from build123d import *

# Parameters (mm, degrees)
ESQUISSE1_R        = 13.55
ESQUISSE1_R_2      = 12.55
BOSS_EXTRU_1_DEPTH = 20
CONG_1_R           = 10
CONG_2_R           = 5


with BuildPart() as part:
    # Esquisse1 → Boss.-Extru.1 (new body)
    with BuildSketch(Plane.XY):
        Circle(ESQUISSE1_R)
        Circle(ESQUISSE1_R_2, mode=Mode.SUBTRACT)
    extrude(amount=BOSS_EXTRU_1_DEPTH)

    # Esquisse2 → Révolution1 (revolve)
    with BuildSketch(Plane(origin=(0, 0, 0), x_dir=(0, 0, -1), z_dir=(1, 0, 0)), mode=Mode.PRIVATE) as r_volution1_sk:
        with BuildLine():
            Line((18.986494144, 0), (0, 0))
            Line((0, 0), (0, -18.986494144))
            ThreePointArc((0, -18.986494144), (13.42547876, -13.42547876), (18.986494144, 0))
        make_face()
    revolve(r_volution1_sk.sketch.rotate(Axis((0, 0, -18.986494144), (0, 0, 1)), 270), axis=Axis((0, 0, -18.986494144), (0, 0, 1)))

    # Congé1
    # the kernel refuses this fillet: 10 mm, written as the material it adds along each edge
    with BuildSketch(Plane(origin=(0, 0, 0), x_dir=(1, 0, 0), z_dir=(0, -1, 0))) as cong_1_piece_1:
        with BuildLine():
            CenterArc((23.55, 8.898000579), CONG_1_R, 180, 62.848132995)
            Line((13.55, 8.898000579), (13.35, 8.898000579))
            Line((13.35, 8.898000579), (13.35, 0))
            Line((13.35, 0), (13.55, -0.2))
            ThreePointArc((13.55, -0.2), (16.268247072, -0.2), (18.895224027, -0.177960012))
            Line((18.895224027, -0.177960012), (18.986494144, 0))
        make_face()
    revolve(axis=Axis((0, 0, 0), (0, 0, 1)))

    # Congé2
    cong_2_edges = [part.edges().sort_by_distance(p)[0] for p in [
        (0, 18.986494144, 0),
    ]]
    fillet(cong_2_edges, radius=CONG_2_R)


solid = part.part
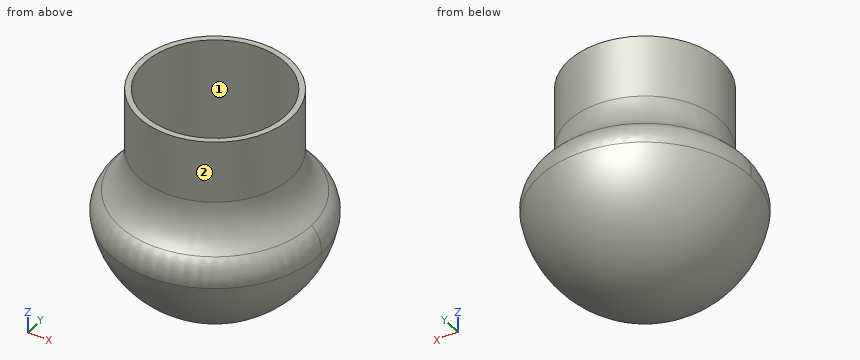
Source: CAD feature listing. Evaluate the final solid. Frame: model axes, mm. Face numbers are marked on the shaded views. Give positions to 0.01 mm unless a question says otherwise; leave off trailing zeros. Write each loop counter-clockwise with the first axis right and the second up, starting at its lowest first coordinate (ties: lowest second). Pieces come first, ordered by that corner, then holes. Notation, with made-up numbers: M -13.5,-20 L 28.5,-20 A25 ccw 28.5,17 Z; hole C 50,71 d1. An arc over 180 degrees is marked long. Return JSON: item names as keys, results as strings. Group by question number.
1) Pin query (flat end, axial travel): P1, Ø8, axis at y = -6.5, z = 9.5, coming from the -X side; P2, Ø12, axis at x = -14, z = -3, coming from the -Y side; P3, Ø10, axis at y = 14, z = 13.5, coming from the -X side. Return the tip coordinate at first contact, or that it passes through.
2) Pull-direction query (Y, two-part tool) for the marked faces 1 and 2; classes: pulls with the +Y half, pulls with the -Y half, needs draft (parallel to the pull), parting line crosses it, or undercut.
3) Cut plane A-A, the plane z = 13. Output: boundary loops of the cut face in (x, y), plus the area to 3 significant figures.
4) Material intervals for line 1 along Y through (x, z) = (0, 9.25); line 2 along Y through (x, z) = (-10, 6); line 3 along Z through (x, y) = (9, -8.5), sorted ascending. Write a range as [from, to].
5) Cut plane B-B, the plane z = -12. Output: boundary loops of the cut face in (x, y), plus the area to 3 significant figures.
Recorded:
{
 "1": {"P1": "stops at x = -13.32", "P2": "stops at y = -16.97", "P3": "stops at x = -10.13"},
 "2": {"face 1": "undercut", "face 2": "parting line crosses it"},
 "3": {"outline": "C 0,0 d27.1; hole C 0,0 d25.1", "area": "82.0 mm²"},
 "4": {"line 1": "y = [-13.55, -12.55], [12.55, 13.55]", "line 2": "y = [-9.77, -7.58], [7.58, 9.77]", "line 3": "z = [-14.4, 0]"},
 "5": {"outline": "C 0,0 d29.43", "area": "680 mm²"}
}
